CAD build for the part. Positions are in the model's coordinates, mm. A direction names the side the tool comes from. Round coordinates to 2 decimals unless told otherwise and drop trailing zeros. Order: outer loops, then holes, each group sorted by start corner. A loop starts at its lowest first (then second) coordinate and runs counter-clockwise, first axis right, second up. Notation, with made-up numbers: (-1.75, -34.5) - (5.25, -34.5) arc R23 cw to (5.25, -3.5) - close; hole circle Ø9 at (37, 39). An arc over 180 degrees is marked (long way). Write item = value, one per line.
from build123d import *

# Parameters (mm, degrees)
F1_DEPTH = 152.4
F3_DEPTH = 76.2
F5_DEPTH = 76.2


with BuildPart() as f1:
    # F0 (on Right) → F1 (new body)
    with BuildSketch(Plane.YZ):
        Polygon((-12.7, 25.4), (-38.1, 25.4), (-38.1, -25.4), (38.1, -25.4), (38.1, 25.4), (12.7, 25.4), (12.7, 12.7), (25.4, 12.7), (25.4, 0), (-25.4, 0), (-25.4, 12.7), (-12.7, 12.7), align=None)
    extrude(amount=F1_DEPTH)

    # F2 (on Front) → F3 (cut)
    with BuildSketch(Plane.XZ):
        Polygon((25.4, -13.421915), (38.1, -25.4), (93.651866, -25.4), (114.3, -25.4), (127, -13.421915), align=None)
    extrude(amount=-F3_DEPTH, mode=Mode.SUBTRACT)

    # F4 (on face) → F5 (cut)
    with BuildSketch(Plane(origin=(0, 0, 0), x_dir=(-1, 0, 0), z_dir=(0, 1, 0))):
        Polygon((-114.3, -25.4), (-38.1, -25.4), (-25.4, -13.421915), (-127, -13.421915), align=None)
    extrude(amount=-F5_DEPTH, mode=Mode.SUBTRACT)


solid = f1.part
(1) Drop flat-ended pins along their axis: pin 1 (10 mm diameter, centred on x = 43.5, y = 16.5, fed in from -Z); pin 2 (1.5 mm diameter, centred on x = 44.5, y = 3, fed in from +Z). Give the stop position or say it passes through.
Solved:
pin_1 = -13.42
pin_2 = 0
(2) Band-saw the part on C-C on x = 36.5. List the corners of the cut face in (y, z).
Solved:
outline = (-38.1, -25.4) - (38.1, -25.4) - (38.1, -23.89) - (-38.1, -23.89) - close; (-38.1, -13.42) - (38.1, -13.42) - (38.1, 25.4) - (12.7, 25.4) - (12.7, 12.7) - (25.4, 12.7) - (25.4, 0) - (-25.4, 0) - (-25.4, 12.7) - (-12.7, 12.7) - (-12.7, 25.4) - (-38.1, 25.4) - close
(3) Pull direction Z, two halves, no side cores. Call faces 6 (the flat face through (75, -25, 25.4)), 7 (the flat face through (75, 25.4, 6)), 8 (the flat face through (75, 38.1, 0)): released by +Z, released by -Z, zero draft, split by the parting line, or undercut.
Solved:
face_6 = released by +Z
face_7 = undercut
face_8 = zero draft
(4) Band-saw the part on D-D on y = 32. List the corners of the cut face in (x, z).
Solved:
outline = (0, -25.4) - (38.1, -25.4) - (25.4, -13.42) - (127, -13.42) - (114.3, -25.4) - (152.4, -25.4) - (152.4, 25.4) - (0, 25.4) - close
(5) Probe line 1 along Y through (x, z) = (57, 11.5); line 2 along Y through (x, z) = (63.5, 13); line 3 along Z through (x, y) = (79, 14). List the from-to ranges inside material, lowest first.
Solved:
line_1 = -38.1 to -25.4, 25.4 to 38.1
line_2 = -38.1 to -12.7, 12.7 to 38.1
line_3 = -13.42 to 0, 12.7 to 25.4
(6) Tool access for faces 1 (the flat face through (75, 12.7, 19)), 2 (the flat face through (75, -19, 12.7)), 3 (the flat face through (75, -38.1, 0)), 4 (the flat face through (75, 1, -13.422)), 5 (the flat face through (19, -1, -25.4)): list every direction of +Z, -Z, +X, -X, +Y, -Y with a clear straight run to the whole face (end or side of a thin tool).
Solved:
face_1 = +Z, +X, -X
face_2 = +X, -X
face_3 = +Z, -Z, +X, -X, -Y
face_4 = +Y, -Y
face_5 = -Z, +X, -X, +Y, -Y
(7) Band-saw the part on A-A on z = 2.5. List the corners of the cut face in (x, y), plus the area to 3 significant figures.
Solved:
outline = (0, -38.1) - (152.4, -38.1) - (152.4, -25.4) - (0, -25.4) - close; (0, 25.4) - (152.4, 25.4) - (152.4, 38.1) - (0, 38.1) - close
area = 3,870 mm²
(8) Band-saw the part on B-B on y = -21.5. List the corners of the cut face in (x, z).
Solved:
outline = (0, -25.4) - (38.1, -25.4) - (25.4, -13.42) - (127, -13.42) - (114.3, -25.4) - (152.4, -25.4) - (152.4, 0) - (0, 0) - close; (0, 12.7) - (152.4, 12.7) - (152.4, 25.4) - (0, 25.4) - close
